```python
from build123d import *

# Parameters (mm, degrees)
ESQUISSE1_R             = 7
BOSS_EXTRU_1_DEPTH      = 25
ENL_V_MAT_EXTRU_1_REACH = 27
ESQUISSE2_R             = 2.5
CHANFREIN1_SIZE         = 0.5
CHANFREIN2_SIZE         = 1
ENL_V_MAT_EXTRU_2_DEPTH = 10
ESQUISSE4_R             = 1.5
ENL_V_MAT_EXTRU_3_DEPTH = 13.361902647


with BuildPart() as part:
    # Esquisse1 → Boss.-Extru.1 (new body)
    with BuildSketch(Plane(origin=(0, 0, 0), x_dir=(1, 0, 0), z_dir=(0, 1, 0))):
        Circle(ESQUISSE1_R)
    extrude(amount=BOSS_EXTRU_1_DEPTH)

    # Esquisse2 → Enlèv. mat.-Extru.1 (cut, up to next)
    with BuildSketch(Plane(origin=(0, 0, 0), x_dir=(-1, 0, 0), z_dir=(0, -1, 0)), mode=Mode.PRIVATE) as enl_v_mat_extru_1_sk1:
        Circle(ESQUISSE2_R)
    enl_v_mat_extru_1_tool1 = extrude(enl_v_mat_extru_1_sk1.sketch, amount=-ENL_V_MAT_EXTRU_1_REACH, mode=Mode.PRIVATE) & part.part
    add(enl_v_mat_extru_1_tool1.solids().sort_by_distance((0, 0, 0))[0], mode=Mode.SUBTRACT)

    # Chanfrein1
    chanfrein1_edges = [part.edges().sort_by_distance(p)[0] for p in [
        (2.5, 0, 0),
    ]]
    chamfer(chanfrein1_edges, length=CHANFREIN1_SIZE)

    # Chanfrein2
    chanfrein2_edges = [part.edges().sort_by_distance(p)[0] for p in [
        (2.5, 25, 0),
    ]]
    chamfer(chanfrein2_edges, length=CHANFREIN2_SIZE)

    # Esquisse3 → Enlèv. mat.-Extru.2 (cut)
    with BuildSketch(Plane(origin=(0, 25, 0), x_dir=(1, 0, 0), z_dir=(0, 1, 0))):
        Polygon((5.361902647, 48.267833041), (5.361902647, 4.5), (5.361902647, -4.5), (5.361902647, -48.267833041), (92.897568728, -48.267833041), (92.897568728, 48.267833041), align=None)
    extrude(amount=-ENL_V_MAT_EXTRU_2_DEPTH, mode=Mode.SUBTRACT)

    # Esquisse4 → Enlèv. mat.-Extru.3 (cut, through all)
    with BuildSketch(Plane(origin=(5.361902647, 0, 0), x_dir=(0, 0, -1), z_dir=(1, 0, 0))):
        with Locations((0, 20)):
            Circle(ESQUISSE4_R)
    extrude(amount=-ENL_V_MAT_EXTRU_3_DEPTH, mode=Mode.SUBTRACT)


solid = part.part
```
The model under review builds one solid part; all positions refer to its coordinate system, in mm. Round coordinates to 2 decimals unless told otherwise and drop trailing zeros. Write each loop counter-clockwise with the first axis right and the second up, starting at its lowest first coordinate (ties: lowest second). Pieces come first, ordered by that corner, then holes.
(1) Insertion check: pin 1 (3 mm diameter, centred on x = -1, y = 11, fed in from -Z); pin 2 (4.5 mm diameter, centred on y = 20.5, z = 0, fed in from +X); pin 3 (3 mm diameter, centred on x = -4, y = 4, fed in from -Z); pin 4 (1 mm diameter, centred on y = 4.5, z = -4.5, fed in from +X). Each pin has a flat end and moves straight along its axis. Give the tip position at first contact, or say it passes through.
(2) Wall thickness on L1, parallel to Z at x = 0, y = 6.5; L2, parallel to Y at x = 4.6, z = 0: over which ranges is each line inside the solid? List them lowest first.
(3) Mouldability with a two-part tool opening along Y and no side actions: class faces 1 (the cylindrical face through (-4.47, 20.07, 1.5)), 2 (the flat face through (5.362, 20, 2)), 3 (the flat face through (6, 15, 0)) as +Y half, -Y half, draft (parallel to the pull), parting line (faces both ways), or undercut.
(4) We need section D-D on y = 20. Give the boundary of the cut face in (x, z).
(5) We need section C-C on y = 3.5. Give the boundary of the cut face in (x, z).
(6) We need section A-A on z = 0. Give the boundary of the cut face in (x, y), and give its area (3 significant figures).
(7) We need section B-B on x = 0. Give the boundary of the cut face in (y, z).
Findings below:
1. pin 1: stops at z = -7
1. pin 2: stops at x = 5.36
1. pin 3: stops at z = -6.54
1. pin 4: stops at x = 5.74
2. L1: z = -7 to -2.5, 2.5 to 7
2. L2: y = 0 to 18.5, 21.5 to 25
3. face 1: undercut
3. face 2: draft
3. face 3: +Y half
4. outline: (-6.84, -1.5) arc R7 ccw to (5.36, -4.5) - (5.36, -1.5) - (2, -1.5) arc R2.5 cw to (-2, -1.5) - close; (-6.84, 1.5) - (-2, 1.5) arc R2.5 cw to (2, 1.5) - (5.36, 1.5) - (5.36, 4.5) arc R7 ccw to start
5. outline: circle Ø14 at (0, 0); hole circle Ø5 at (0, 0)
6. outline: (-7, 0) - (-3, 0) - (-2.5, 0.5) - (-2.5, 18.5) - (-7, 18.5) - close; (-7, 21.5) - (-2.5, 21.5) - (-2.5, 24) - (-3.5, 25) - (-7, 25) - close; (2.5, 0.5) - (3, 0) - (7, 0) - (7, 15) - (5.36, 15) - (5.36, 18.5) - (2.5, 18.5) - close; (2.5, 21.5) - (5.36, 21.5) - (5.36, 25) - (3.5, 25) - (2.5, 24) - close
6. area: 185 mm2
7. outline: (0, -7) - (25, -7) - (25, -3.5) - (24, -2.5) - (0.5, -2.5) - (0, -3) - close; (0, 3) - (0.5, 2.5) - (24, 2.5) - (25, 3.5) - (25, 7) - (0, 7) - close
